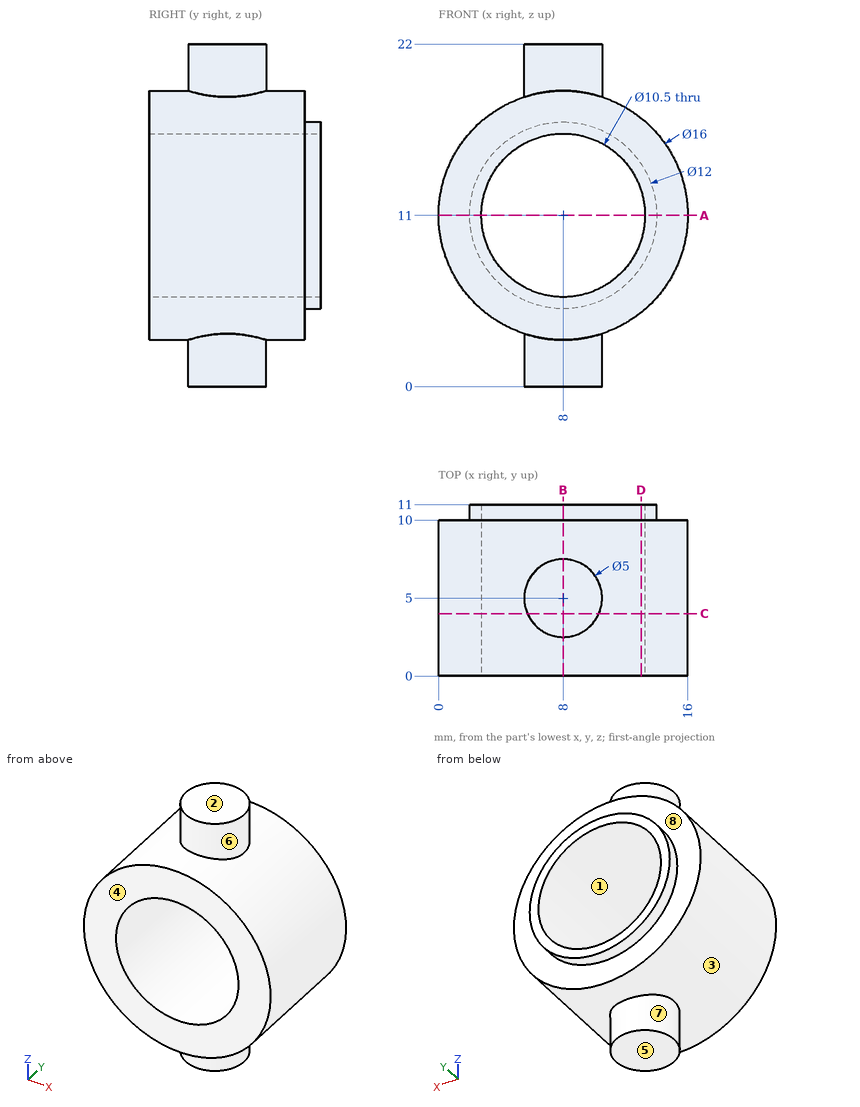
Design review of the part shown in the three views and the two pictorial views. Dimensions are in mm from the part's minimum x, y and z. A direction names the side the tool comes from. Round coordinates to 2 decimals unless told otherwise and drop trailing zeros. Order: outer loops, then holes, each group sorted by start corner. A loop starts at its lowest first (then second) coordinate and runs counter-clockwise, first axis right, second up.
Item 1: Add section C-C, the plane y = 4. State the section outline as (x, z) points, and give its area (3 significant figures).
Working result:
outline: (5.71, 0) - (10.29, 0) - (10.29, 3.34) arc R8 ccw to (10.29, 18.66) - (10.29, 22) - (5.71, 22) - (5.71, 18.66) arc R8 ccw to (5.71, 3.34) - close; hole circle Ø10.5 at (8, 11)
area: 143 mm2
Item 2: Machinability: for the marked faces 4, 5, 6, 7 and 8, which of the approach directions +Z, -Z, +X, -X, +Y, -Y give a long, thin tool a straight path to every point of the face, cutting with its end or side? Answer none if there is none.
Working result:
face 4: +Z, -Z, +X, -X, -Y
face 5: -Z, +X, -X, +Y, -Y
face 6: +Z
face 7: -Z
face 8: +Y
Item 3: To check wall thickness, follow probe 1 along X at (y, z) = (3, 11); probe 2 along X at (y, z) = (9.5, 9.5); probe 3 along Z at (x, y) = (6.75, 4). State the ranges of each line that lie inside material, in increasing order.
Working result:
probe 1: x = 0 to 2.75, 13.25 to 16
probe 2: x = 0.14 to 2.97, 13.03 to 15.86
probe 3: z = 0 to 5.9, 16.1 to 22
Item 4: Add section D-D, the plane x = 13. State the section outline as (y, z) points (3 decimals), and give its area (3 significant figures).
Working result:
outline: (0, 4.755) - (10, 4.755) - (10, 7.683) - (11, 7.683) - (11, 9.399) - (0, 9.399) - close; (0, 12.601) - (11, 12.601) - (11, 14.317) - (10, 14.317) - (10, 17.245) - (0, 17.245) - close
area: 96.3 mm2
Item 5: For pin 1 (4 mm diameter, centred on y = 9, z = 6, fed in from -X); pin 2 (1 mm diameter, centred on y = 5, z = 8, fed in from +X); pin 3 (9.5 mm diameter, centred on x = 8, z = 11, fed in from +Y); pin 4 (2 mm diameter, centred on x = 10, y = 9, fed in from -Z), all flat-tipped, find the tip position at first contact; note any pin that passes through.
Working result:
pin 1: stops at x = 0.58
pin 2: stops at x = 15.6
pin 3: passes through
pin 4: stops at z = 3.06
Item 6: Draft analysis for pull direction X (two halves, no side actions). For the marked faces 1, 2 and 3, state which applies: released by +X, released by -X, zero draft, split by the parting line, or undercut.
Working result:
face 1: undercut
face 2: zero draft
face 3: split by the parting line
Item 7: Add section A-A, the plane z = 11. State the section outline as (x, y) points, and give its area (3 significant figures).
Working result:
outline: (0, 0) - (2.75, 0) - (2.75, 11) - (2, 11) - (2, 10) - (0, 10) - close; (13.25, 0) - (16, 0) - (16, 10) - (14, 10) - (14, 11) - (13.25, 11) - close
area: 56.5 mm2
Item 8: Add section B-B, the plane x = 8. State the section outline as (y, z) points, and give its area (3 significant figures).
Working result:
outline: (0, 3) - (2.5, 3) - (2.5, 0) - (7.5, 0) - (7.5, 3) - (10, 3) - (10, 5) - (11, 5) - (11, 5.75) - (0, 5.75) - close; (0, 16.25) - (11, 16.25) - (11, 17) - (10, 17) - (10, 19) - (7.5, 19) - (7.5, 22) - (2.5, 22) - (2.5, 19) - (0, 19) - close
area: 86.5 mm2
